```python
from build123d import *

# Parameters (mm, degrees)
SKETCH1_R           = 9.975
BOSS_EXTRUDE1_DEPTH = 2.5
SKETCH3_W           = 24.73
SKETCH3_H           = 35
BOSS_EXTRUDE4_DEPTH = 2.5
SKETCH3_5_W         = 32.73
SKETCH3_5_H         = 43
SKETCH3_5_W_2       = 24.73
SKETCH3_5_H_2       = 35
BOSS_EXTRUDE5_DEPTH = 21.4
SKETCH4_W           = 5.2
SKETCH4_H           = 1.1
SKETCH4_W_2         = 3.2
SKETCH4_H_2         = 1.5
BOSS_EXTRUDE6_DEPTH = 18.9
SKETCH6_W           = 18.33
SKETCH6_H           = 1.5
BOSS_EXTRUDE7_DEPTH = 5.3
SKETCH2_R           = 1.6
CUT_EXTRUDE1_DEPTH  = 37


with BuildPart() as part:
    # Sketch1 → Boss-Extrude1 (new body)
    with BuildSketch(Plane.XY):
        Circle(SKETCH1_R)
    extrude(amount=BOSS_EXTRUDE1_DEPTH)

    # Sketch3 → Boss-Extrude4 (add)
    with BuildSketch(Plane(origin=(0, 0, 0), x_dir=(-1, 0, 0), z_dir=(0, 0, -1))):
        Rectangle(SKETCH3_W, SKETCH3_H)
    extrude(amount=BOSS_EXTRUDE4_DEPTH)

    # Sketch3<5> → Boss-Extrude5 (add)
    with BuildSketch(Plane(origin=(0, 0, 0), x_dir=(-1, 0, 0), z_dir=(0, 0, -1))):
        Rectangle(SKETCH3_5_W, SKETCH3_5_H)
        Rectangle(SKETCH3_5_W_2, SKETCH3_5_H_2, mode=Mode.SUBTRACT)
    extrude(amount=BOSS_EXTRUDE5_DEPTH)

    # Sketch4 → Boss-Extrude6 (add)
    with BuildSketch(Plane(origin=(0, 0, -2.5), x_dir=(-1, 0, 0), z_dir=(0, 0, -1))):
        with Locations((9.765, 16.95)):
            Rectangle(SKETCH4_W, SKETCH4_H)
        with Locations((-9.765, 16.95)):
            Rectangle(SKETCH4_W, SKETCH4_H)
        with Locations((10.765, -16.75)):
            Rectangle(SKETCH4_W_2, SKETCH4_H_2)
        with Locations((-10.765, -16.75)):
            Rectangle(SKETCH4_W_2, SKETCH4_H_2)
    extrude(amount=BOSS_EXTRUDE6_DEPTH)

    # Sketch6 → Boss-Extrude7 (add)
    with BuildSketch(Plane(origin=(0, 0, -2.5), x_dir=(-1, 0, 0), z_dir=(0, 0, -1))):
        with Locations((0, -16.75)):
            Rectangle(SKETCH6_W, SKETCH6_H)
    extrude(amount=BOSS_EXTRUDE7_DEPTH)

    # Sketch2 → Cut-Extrude1 (cut)
    with BuildSketch(Plane.XY.offset(2.5)):
        with Locations((7, 0)):
            Circle(SKETCH2_R)
        with Locations((0, -7)):
            Circle(SKETCH2_R)
        with Locations((-7, 0)):
            Circle(SKETCH2_R)
        with Locations((0, 7)):
            Circle(SKETCH2_R)
    extrude(amount=-CUT_EXTRUDE1_DEPTH, mode=Mode.SUBTRACT)


solid = part.part
```
Could you check a few things on this model? Use its own coordinates, in mm. A direction names the side the tool comes from. Give positions to 0.01 mm unless a question says otherwise; leave off trailing zeros. Write each loop counter-clockwise with the first axis right and the second up, starting at its lowest first coordinate (ties: lowest second). Pieces come first, ordered by that corner, then holes. Notation, with made-up numbers: (41.25, 33) - (88.25, 33) arc R17 ccw to (88.25, 52) - close; hole circle Ø8 at (-20, 59). An arc over 180 degrees is marked (long way). One line per item, written item: value. Start each with the question number.
Item 1: Imagine slicing it at C-C, the plane y = 7. List the corners of the cut face in (x, z) for me (3 decimals), and give its area (3 significant figures).
Item 2: I'm going to push flat-ended pins straight in: pin 1 (0.8 mm diameter, centred on x = -3, y = -17, fed in from -Z); pin 2 (3 mm diameter, centred on x = 5, y = -12.5, fed in from +Z); pin 3 (4 mm diameter, centred on x = 7, y = 0, fed in from -Z). Where does each tip first touch, or does it pass through?
Item 3: Which directions (+Z, -Z, +X, -X, +Y, -Y) give clear straight access to the entire face, cutting with the end or side of a thin tool? Please do faces 1 (the face through (4, 10, 0)), 2 (the face through (0, 21.5, -11)), 3 (the face through (-10, 16.4, -12)).
Item 4: Please list where these lines run through material, in increasing order: line 1 (X direction, y = -13, z = -13) (3 decimals); line 2 (Y direction, x = 0, z = -0.95); line 3 (Y direction, x = -2, z = -6.25). Write a range as from..to.
Item 5: Imagine slicing it at B-B, the plane z = -15.5. List the corners of the cut face in (x, y) for me (3 decimals), and give its area (3 significant figures).
Item 6: Imagine slicing it at D-D, the plane y = 0. List the corners of the cut face in (x, z) for me (3 decimals).
Item 7: Imagine slicing it at A-A, the plane x = 0. List the corners of the cut face in (y, z) for me (3 decimals), and give its area (3 significant figures).
Item 8: If we mould it in two halves opening along Y, with no side actions, what happens to faces 4 (the face through (9.514, 2.996, 1.232)), 5 (the face through (7.165, 17, -12)), 6 (the face through (-16.365, 0, -11)), 7 (the face through (-0.35, -8.56, 0.04))? For each: +Y half, -Y half, draft (parallel to the pull), parting line (faces both ways), or undercut.
Geometry says:
1. outline: (-16.365, -21.4) - (-12.365, -21.4) - (-12.365, -2.5) - (-1.6, -2.5) - (-1.6, 2.5) - (-7.106, 2.5) - (-7.106, 0) - (-16.365, 0) - close; (1.6, -2.5) - (12.365, -2.5) - (12.365, -21.4) - (16.365, -21.4) - (16.365, 0) - (7.106, 0) - (7.106, 2.5) - (1.6, 2.5) - close
1. area: 253 mm^2
2. pin 1: z = -7.8
2. pin 2: z = 0
2. pin 3: z = -2.5
3. face 1: +Z
3. face 2: +Z, -Z, +X, -X, +Y
3. face 3: -Z
4. line 1: -16.365..-12.365, 12.365..16.365
4. line 2: -21.5..-8.6, -5.4..5.4, 8.6..21.5
4. line 3: -21.5..-16, 17.5..21.5
5. outline: (-16.365, -21.5) - (16.365, -21.5) - (16.365, 21.5) - (-16.365, 21.5) - close; hole (-12.365, -16) - (-9.165, -16) - (-9.165, -17.5) - (9.165, -17.5) - (9.165, -16) - (12.365, -16) - (12.365, 16.4) - (7.165, 16.4) - (7.165, 17.5) - (-7.165, 17.5) - (-7.165, 16.4) - (-12.365, 16.4) - close
5. area: 563 mm^2
6. outline: (-16.365, -21.4) - (-12.365, -21.4) - (-12.365, -2.5) - (-8.6, -2.5) - (-8.6, 2.5) - (-9.975, 2.5) - (-9.975, 0) - (-16.365, 0) - close; (-5.4, -2.5) - (5.4, -2.5) - (5.4, 2.5) - (-5.4, 2.5) - close; (8.6, -2.5) - (12.365, -2.5) - (12.365, -21.4) - (16.365, -21.4) - (16.365, 0) - (9.975, 0) - (9.975, 2.5) - (8.6, 2.5) - close
7. outline: (-21.5, -21.4) - (-17.5, -21.4) - (-17.5, -7.8) - (-16, -7.8) - (-16, -2.5) - (-8.6, -2.5) - (-8.6, 2.5) - (-9.975, 2.5) - (-9.975, 0) - (-21.5, 0) - close; (-5.4, -2.5) - (5.4, -2.5) - (5.4, 2.5) - (-5.4, 2.5) - close; (8.6, -2.5) - (17.5, -2.5) - (17.5, -21.4) - (21.5, -21.4) - (21.5, 0) - (9.975, 0) - (9.975, 2.5) - (8.6, 2.5) - close
7. area: 285 mm^2
8. face 4: parting line
8. face 5: undercut
8. face 6: draft
8. face 7: undercut
